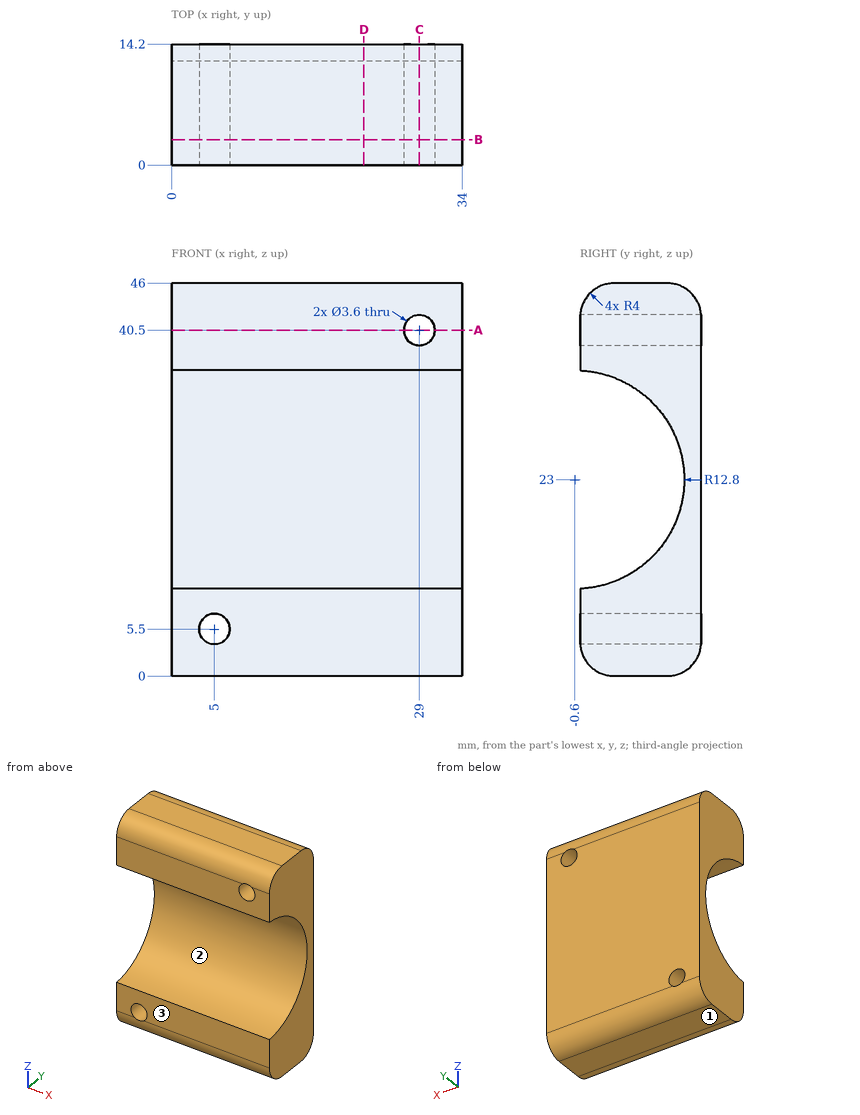
Answer from the drawing. Dimensions are ordinates in mm from the lowest x, y and z of the part. Round coordinates to 2 decimals unless told otherwise and drop trailing zeros. Loops run counter-clockwise (first coordinate to the right, second up) from the corner with the lowest first, then second, coordinate; pieces in that order, holes last. Notation, with made-up numbers: M 61.25,22.5 L 78.25,22.5 A21 cw 78.25,39.5 Z; hole C 22,22 d11. An arc over 180 degrees is marked long. One line per question, with ' | ' between items. Start each with the question number.
(1) A cutting plane is placed at D-D on x = 22.5. Write down the section's boundary in (y, z).
(2) A flat-ended cylindrical pin translates along its axis: pin 1 Ø3 at (x, z) = (29, 40.5) entering from +Y. Find the tip coordinate at first contact, or state that the pin passes through.
(3) A cutting plane is placed at A-A on z = 40.5. Write down the section's boundary in (x, y), plus the area to 3 significant figures.
(4) For a pull along Z with two mould halves and no side action, classify the marked faces 1, 2 and 3 as released by +Z, released by -Z, zero draft, split by the parting line, or undercut.
(5) Find the intervals of material crossed by line 1 (X direction, y = 11, z = 5.5); line 2 (X direction, y = 6, z = 40.5); line 3 (Z direction, x = 29, y = 10.5), in increasing order.
(6) A cutting plane is placed at B-B on y = 3. Write down the section's boundary in (x, z).
(7) A cutting plane is placed at C-C on x = 29. Write down the section's boundary in (y, z), plus the area to 3 significant figures.
Geometry check:
1) outline: M 0,4 A4 ccw 4,0 L 10.2,0 A4 ccw 14.2,4 L 14.2,42 A4 ccw 10.2,46 L 4,46 A4 ccw 0,42 L 0,35.79 A12.8 cw 0,10.21 Z
2) pin 1: passes through
3) outline: M 0,0 L 27.2,0 L 27.2,14.2 L 0,14.2 Z; M 30.8,0 L 34,0 L 34,14.2 L 30.8,14.2 Z | area: 432 mm²
4) face 1: released by -Z | face 2: undercut | face 3: zero draft
5) line 1: x = 0 to 3.2, 6.8 to 34 | line 2: x = 0 to 27.2, 30.8 to 34 | line 3: z = 0.01 to 16.63, 29.37 to 38.7, 42.3 to 45.99
6) outline: M 0,0.13 L 34,0.13 L 34,10.72 L 0,10.72 Z; M 0,35.28 L 34,35.28 L 34,45.87 L 0,45.87 Z; hole C 5,5.5 d3.6; hole C 29,40.5 d3.6
7) outline: M 0,4 A4 ccw 4,0 L 10.2,0 A4 ccw 14.2,4 L 14.2,38.7 L 0,38.7 L 0,35.79 A12.8 cw 0,10.21 Z; M 0.01,42.3 L 14.19,42.3 A4 ccw 10.2,46 L 4,46 A4 ccw Z | area: 346 mm²
